```python
from build123d import *

# Parameters (mm, degrees)
EXTRUDE_1_DEPTH          = 26
CUT_EXTRUDE_1_DEPTH      = 249.953347952
CUT_EXTRUDE_1_DEPTH_BACK = 249.953347952
SKETCH_2_R               = 1.5
FILLET_1_R               = 0.5
CHAMFER_1_SIZE           = 0.5


with BuildPart() as part:
    # 草图1 → 凸台-拉伸1 (new body)
    with BuildSketch(Plane.XY):
        with BuildLine():
            Line((-212.180704616, 127.029942007), (-212.520971413, 110.249281361))
            Line((-212.520971413, 110.249281361), (-176.528370185, 109.519447931))
            ThreePointArc((-176.528370185, 109.519447931), (-196.295218168, 114.323361589), (-212.180704616, 127.029942007))
        make_face()
    extrude(amount=EXTRUDE_1_DEPTH)

    # 草图2 → 切除-拉伸1 (cut, two sides: drawn at the far end of the back side and taken through both)
    with BuildSketch(Plane(origin=(0, 0, 0), x_dir=(-1, 0, 0), z_dir=(0, 0, -1)).offset(-CUT_EXTRUDE_1_DEPTH_BACK)):
        with Locations((200.041202679, 114.05266186)):
            Circle(SKETCH_2_R)
    extrude(amount=CUT_EXTRUDE_1_DEPTH + CUT_EXTRUDE_1_DEPTH_BACK, mode=Mode.SUBTRACT)

    # 圆角1
    fillet_1_edges = [part.edges().sort_by_distance(p)[0] for p in [
        (-212.520971413, 110.249281361, 13),
        (-176.528370185, 109.519447931, 13),
        (-212.180704616, 127.029942007, 13),
    ]]
    fillet(fillet_1_edges, radius=FILLET_1_R)

    # 倒角1
    chamfer_1_edges = [part.edges().sort_by_distance(p)[0] for p in [
        (-199.945178972, 116.321228968, 26),
        (-199.945178972, 116.321228968, 0),
        (-199.121405734, 109.977574103, 0),
        (-212.359389005, 118.217909462, 0),
        (-212.371585967, 110.392728938, 0),
        (-211.876239308, 126.147365712, 0),
        (-185.71538147, 110.154529202, 0),
        (-199.121405734, 109.977574103, 26),
        (-212.359389005, 118.217909462, 26),
        (-212.371585967, 110.392728938, 26),
        (-211.876239308, 126.147365712, 26),
        (-185.71538147, 110.154529202, 26),
    ]]
    chamfer(chamfer_1_edges, length=CHAMFER_1_SIZE)


solid = part.part
```
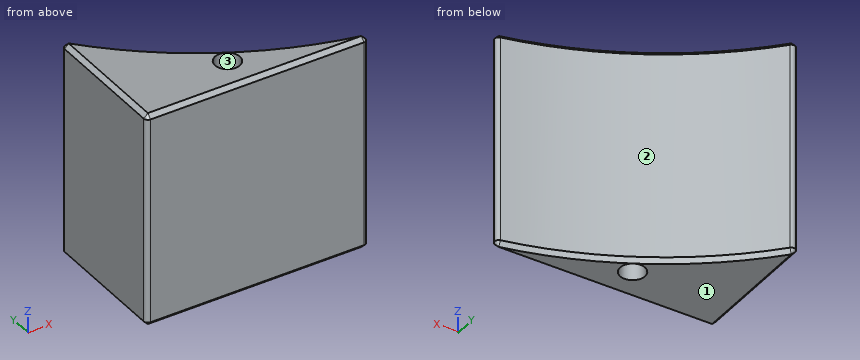
The listing builds one solid part. Answer for the finished solid, in the listing's coordinates (mm). Face numbers are marked on the shaded views. Give positions to 0.01 mm unless a question says otherwise; leave off trailing zeros. Order: outer loops, then holes, each group sorted by start corner. A loop starts at its lowest first (then second) coordinate and runs counter-clockwise, first axis right, second up.
1) Determine the mould class of the marked faces 1, 2 and 3 for opening direction X: pulls with the +X half, pulls with the -X half, needs draft (parallel to the pull), parting line crosses it, or undercut.
Reported:
face 1: needs draft
face 2: pulls with the +X half
face 3: undercut
2) Consider line 1 along X through (y, z) = (121.75, 3.75); line 2 along Y through (x, z) = (-187.25, 24.75); line 3 along X through (y, z) = (123.25, 1.5). Determine where each line is inside the solid, lowest interval first.
Reported:
line 1: x = -212.29 to -207.21
line 2: y = 109.74 to 110.98
line 3: x = -212.26 to -208.78
3) Given P1, Ø6, axis at y = 116, z = 15, coming from the -X side; P2, Ø6, axis at x = -191.5, z = 15.5, coming from the -Y side; P3, Ø4, axis at x = -194, z = 22, coming from the +Y side, each flat-ended and moving along its own axis, determine where each tip first touches the part or whether it passes through.
Reported:
P1: stops at x = -212.47
P2: stops at y = 109.76
P3: stops at y = 114.18
4) Find section A-A on z = 19. Write down the section's boundary in (x, y).
Reported:
outline: (-212.51, 110.75) arc R0.5 ccw to (-212.02, 110.24) - (-186.22, 109.72) arc R0.5 ccw to (-186.1, 110.7) arc R47 cw to (-211.33, 126) arc R0.5 ccw to (-212.21, 125.69) - close; hole circle Ø3 at (-200.04, 114.05)
